Work out the finished part from the listing and answer in its coordinate system (mm). A direction names the side the tool comes from. Round coordinates to 2 decimals unless told otherwise and drop trailing zeros. Order: outer loops, then holes, each group sorted by start corner. A loop starts at its lowest first (then second) coordinate and runs counter-clockwise, first axis right, second up. Notation, with made-up numbers: (-6.5, 54) - (-0.5, 54) arc R12 ccw to (-0.5, 74) - close; hole circle Ø6 at (65.5, -38). An arc over 180 degrees is marked (long way). Use one line per item in the form item = value. Start each with the question number.
Q1. The part is cut by section B-B on x = 9.45. Determine the outline of the cut face in (y, z), plus the area to 3 significant figures.
Q2. For a pull along X with two mould halves and no side action, classify faces 1 (the cylindrical face through (16.12, 1.08, 7.26)), 2 (the cylindrical face through (13.65, 6.57, 1.08)), 3 (the flat face through (0, 5, 1)), 4 (the flat face through (9, 5, 0)) as +X half, -X half, draft (parallel to the pull), parting line (faces both ways), or undercut.
Q3. The part is cut by section D-D on z = 5.7. Determine the outline of the cut face in (x, y).
Q4. The part is cut by section C-C on y = 1.5. Determine the outline of the cut face in (x, z), plus the area to 3 significant figures.
Q5. The part is cut by section A-A on y = 6.5. Determine the outline of the cut face in (x, z).
Q6. Find the intervals of material crossed by line 1 (Y direction, x = 15.15, z = 1.35); line 2 (X direction, y = 1.05, z = 5.7); line 3 (Z direction, x = 15, y = 3), in increasing order. Write a range as [from, to].
Q7. Given P1, Ø4, axis at y = 5.5, z = 9, coming from the +X side; P2, Ø3.5, axis at x = 15.15, y = 6.5, coming from the +Z side, each flat-ended and moving along its own axis, determine where each tip first touches the part or whether it passes through.
Q8. Which of the six approach directions +Z, -Z, +X, -X, +Y, -Y give full straight-line access (tool end or side, diameter ignored) to faces 5 (the flat face through (9, 6, 2.2)), 6 (the flat face through (18.9, 5, 1))?
from build123d import *

# Parameters (mm, degrees)
SKETCH1_R           = 1.5
BOSS_EXTRUDE1_DEPTH = 2.2
SKETCH2_W           = 18.9
SKETCH2_H           = 2.2
BOSS_EXTRUDE2_DEPTH = 7.7
SKETCH3_R           = 1.5
CUT_EXTRUDE1_DEPTH  = 2.2


with BuildPart() as part:
    # Sketch1 → Boss-Extrude1 (new body)
    with BuildSketch(Plane.XY):
        with BuildLine():
            Line((0, 0), (18.9, 0))
            Line((18.9, 0), (18.9, 8.1))
            ThreePointArc((18.9, 8.1), (18.460660172, 9.160660172), (17.4, 9.6))
            Line((17.4, 9.6), (1.5, 9.6))
            ThreePointArc((1.5, 9.6), (0.439339828, 9.160660172), (0, 8.1))
            Line((0, 8.1), (0, 0))
        make_face()
        with Locations((3.75, 6.5)):
            Circle(SKETCH1_R, mode=Mode.SUBTRACT)
        with Locations((15.15, 6.5)):
            Circle(SKETCH1_R, mode=Mode.SUBTRACT)
    extrude(amount=BOSS_EXTRUDE1_DEPTH)

    # Sketch2 → Boss-Extrude2 (add)
    with BuildSketch(Plane.XY.offset(2.2)):
        with Locations((9.45, 1.1)):
            Rectangle(SKETCH2_W, SKETCH2_H)
    extrude(amount=BOSS_EXTRUDE2_DEPTH)

    # Sketch3 → Cut-Extrude1 (cut)
    with BuildSketch(Plane.XZ):
        with BuildLine():
            Line((0, 9.9), (0, 0.65))
            ThreePointArc((0, 0.65), (2.709262274, 7.190737726), (9.25, 9.9))
            Line((9.25, 9.9), (0, 9.9))
        make_face()
        with BuildLine():
            Line((18.9, 9.9), (9.65, 9.9))
            ThreePointArc((9.65, 9.9), (16.190737726, 7.190737726), (18.9, 0.65))
            Line((18.9, 0.65), (18.9, 9.9))
        make_face()
        with Locations(Location((9.45, 5.7, 0), (0, 0, 270))):
            Circle(SKETCH3_R)
    extrude(amount=-CUT_EXTRUDE1_DEPTH, mode=Mode.SUBTRACT)


solid = part.part
Found:
q1.outline = (0, 0) - (9.6, 0) - (9.6, 2.2) - (2.2, 2.2) - (2.2, 4.2) - (0, 4.2) - close; (0, 7.2) - (2.2, 7.2) - (2.2, 9.9) - (0, 9.9) - close
q1.area = 31.5 mm²
q2.face_1 = +X half
q2.face_2 = undercut
q2.face_3 = -X half
q2.face_4 = draft
q3.outline = (1.5, 0) - (7.95, 0) - (7.95, 2.2) - (1.5, 2.2) - close; (10.95, 0) - (17.4, 0) - (17.4, 2.2) - (10.95, 2.2) - close
q4.outline = (0, 0) - (18.9, 0) - (18.9, 0.65) arc R9.25 ccw to (9.65, 9.9) - (9.25, 9.9) arc R9.25 ccw to (0, 0.65) - close; hole circle Ø3 at (9.45, 5.7)
q4.area = 143 mm²
q5.outline = (0, 0) - (2.25, 0) - (2.25, 2.2) - (0, 2.2) - close; (5.25, 0) - (13.65, 0) - (13.65, 2.2) - (5.25, 2.2) - close; (16.65, 0) - (18.9, 0) - (18.9, 2.2) - (16.65, 2.2) - close
q6.line_1 = [0, 5], [8, 9.6]
q6.line_2 = [1.5, 7.95], [10.95, 17.4]
q6.line_3 = [0, 2.2]
q7.P1 = through
q7.P2 = 2.2
q8.face_5 = +Z, +X, -X, +Y
q8.face_6 = +Z, -Z, +X, +Y, -Y
